The listing builds one solid part. Answer for the finished solid, in the listing's coordinates (mm). Face numbers are marked on the shaded views. Give positions to 0.01 mm unless a question says otherwise; leave off trailing zeros. Order: outer loops, then holes, each group sorted by start corner. A loop starts at its lowest first (then second) coordinate and runs counter-clockwise, first axis right, second up.
```python
from build123d import *

# Parameters (mm, degrees)
BOSS_EXTRUDE1_DEPTH = 5.9944
SKETCH2_R           = 4.7625
CUT_EXTRUDE1_DEPTH  = 68.534353797
SKETCH3_R           = 2.286
CUT_EXTRUDE2_DEPTH  = 68.534353797
SKETCH4_W           = 50.8
SKETCH4_H           = 50.8
BOSS_EXTRUDE2_DEPTH = 5.9944
CHAMFER1_SIZE       = 6.35


with BuildPart() as part:
    # Sketch1 → Boss-Extrude1 (new body)
    with BuildSketch(Plane.XY):
        Polygon((0, 0), (-38.1, 0), (-38.1, 6.35), (-44.0944, 6.35), (-44.0944, 19.05), (-38.1, 19.05), (-38.1, 31.75), (-44.0944, 31.75), (-44.0944, 44.45), (-38.1, 44.45), (-38.1, 50.8), (0, 50.8), (0, 44.45), (5.9944, 44.45), (5.9944, 31.75), (0, 31.75), (0, 19.05), (5.9944, 19.05), (5.9944, 6.35), (0, 6.35), align=None)
    extrude(amount=BOSS_EXTRUDE1_DEPTH)

    # Sketch2 → Cut-Extrude1 (cut, through all)
    with BuildSketch(Plane(origin=(0, 0, 0), x_dir=(-1, 0, 0), z_dir=(0, 0, -1))):
        with Locations((19.05, 31.75)):
            Circle(SKETCH2_R)
    extrude(amount=-CUT_EXTRUDE1_DEPTH, mode=Mode.SUBTRACT)

    # Sketch3 → Cut-Extrude2 (cut, through all)
    with BuildSketch(Plane.XY.offset(5.9944)):
        with Locations((-19.05, 19.05)):
            Circle(SKETCH3_R)
        with Locations((-19.05, 6.35)):
            Circle(SKETCH3_R)
    extrude(amount=-CUT_EXTRUDE2_DEPTH, mode=Mode.SUBTRACT)

    # Sketch4 → Boss-Extrude2 (add)
    with BuildSketch(Plane.XY.offset(5.9944)):
        with Locations((-19.05, -25.4)):
            Rectangle(SKETCH4_W, SKETCH4_H)
    extrude(amount=-BOSS_EXTRUDE2_DEPTH)

    # Chamfer1
    chamfer1_edges = [part.edges().sort_by_distance(p)[0] for p in [
        (6.35, 0, 2.9972),
        (6.35, -50.8, 2.9972),
        (-44.45, -50.8, 2.9972),
        (-44.45, 0, 2.9972),
    ]]
    chamfer(chamfer1_edges, length=CHAMFER1_SIZE - 0.0001)  # a hair under: the kernel refuses the full size


solid = part.part
```
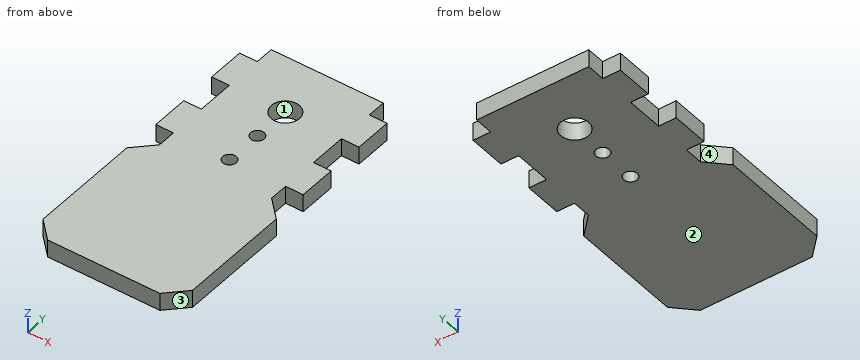
1) Given P1, Ø2, axis at y = 21, z = 1, coming from the +X side; P2, Ø3, axis at x = -40, z = 3.5, coming from the -Y side; P3, Ø1.8, axis at x = -41.5, z = 2.5, coming from the +Y side, each flat-ended and moving along its own axis, determine where each tip first touches the part or whether it passes through.
Geometry says:
P1: stops at x = 0
P2: stops at y = -50.4
P3: stops at y = 44.45
2) For a pull along Y with two mould halves and no side action, classify the marked faces 1, 2, 3 and 4 as +Y half, -Y half, draft (parallel to the pull), parting line (faces both ways), or undercut.
Geometry says:
face 1: undercut
face 2: draft
face 3: -Y half
face 4: undercut
3) Straight lines are drawn through the part: probe 1 along Y at (x, z) = (-19.05, 1.35); probe 2 along Y at (x, z) = (-40, 2.9); probe 3 along Y at (x, z) = (-39, 4). For each, find the intervals that lie inside material, in ascending order.
Geometry says:
probe 1: y = -50.8 to 4.06, 8.64 to 16.76, 21.34 to 26.99, 36.51 to 50.8
probe 2: y = -48.9 to -1.9, 6.35 to 19.05, 31.75 to 44.45
probe 3: y = -49.9 to -0.9, 6.35 to 19.05, 31.75 to 44.45
4) Find section A-A (x = -19.05). Write down the section's boundary in (y, z).
Geometry says:
outline: (-50.8, 0) - (4.06, 0) - (4.06, 5.99) - (-50.8, 5.99) - close; (8.64, 0) - (16.76, 0) - (16.76, 5.99) - (8.64, 5.99) - close; (21.34, 0) - (26.99, 0) - (26.99, 5.99) - (21.34, 5.99) - close; (36.51, 0) - (50.8, 0) - (50.8, 5.99) - (36.51, 5.99) - close
5) Find section C-C (y = 1.5). Write down the section's boundary in (x, z), then the cut area to 3 significant figures.
Geometry says:
outline: (-38.1, 0) - (0, 0) - (0, 5.99) - (-38.1, 5.99) - close
area: 228 mm2
6) Find section B-B (z = 3.65). Count the separate pieces of the cut face and the enclosed holes in it, then the cut area to 3 significant figures.
Geometry says:
separate pieces: 1
enclosed holes: 3
area: 4,640 mm2
